from build123d import *

# Parameters (mm, degrees)
SKETCH_13_W                      = 40
SKETCH_13_H                      = 5
SM_BASE_FLANGE_1_DEPTH           = 18
SM_EDGE_FLANGE_1_STRIP_W         = 23.4732
SM_EDGE_FLANGE_1_STRIP_H         = 5
SM_EDGE_FLANGE_1_STRIP_CUT_DEPTH = 40
SM_EDGE_FLANGE_1_DEPTH           = 40
SKETCH_26_R                      = 1.5
CUT_EXTRUDE_1_DEPTH              = 81.956778592
FILLET_1_R                       = 3
SKETCH_32_R                      = 3.3
CUT_EXTRUDE_4_DEPTH              = 1


# Sheet-metal steps are written as plain solids
with BuildPart() as part:
    # 草图13 → 基体-法兰1 (new body)
    with BuildSketch(Plane.XY):
        with Locations((0, -2.5)):
            Rectangle(SKETCH_13_W, SKETCH_13_H)
    extrude(amount=SM_BASE_FLANGE_1_DEPTH)

    # 边线-法兰1 strip (across the edge) → 边线-法兰1 strip cut (cut)
    with BuildSketch(Plane(origin=(-20, 0, 18), x_dir=(0, 0, -1), z_dir=(1, 0, 0))):
        with Locations((-10, -2.5)):
            Rectangle(SM_EDGE_FLANGE_1_STRIP_W, SM_EDGE_FLANGE_1_STRIP_H)
    extrude(amount=SM_EDGE_FLANGE_1_STRIP_CUT_DEPTH, mode=Mode.SUBTRACT)

    # 边线-法兰1 section (across the edge) → 边线-法兰1 (add)
    with BuildSketch(Plane(origin=(-20, 0, 18), x_dir=(0, 0, -1), z_dir=(1, 0, 0))):
        with BuildLine():
            Line((-5, 1.7366), (-5, 70))
            Line((-5, 70), (0, 70))
            Line((0, 70), (0, 1.7366))
            ThreePointArc((0, 1.7366), (0.508638364, 0.508638364), (1.7366, 0))
            Line((1.7366, 0), (1.7366, -5))
            ThreePointArc((1.7366, -5), (-3.026895542, -3.026895542), (-5, 1.7366))
        make_face()
    extrude(amount=SM_EDGE_FLANGE_1_DEPTH)

    # 草图26 → 切除-拉伸1 (cut, through all)
    with BuildSketch(Plane.XZ.offset(5)):
        with Locations(Location((-13.7, 5.5, 0), (0, 0, 270))):
            Circle(SKETCH_26_R)
        with Locations(Location((13.7, 5.5, 0), (0, 0, 270))):
            Circle(SKETCH_26_R)
    extrude(amount=-CUT_EXTRUDE_1_DEPTH, mode=Mode.SUBTRACT)

    # 圆角1
    fillet_1_edges = [part.edges().sort_by_distance(p)[0] for p in [
        (-20, -2.5, 0),
        (20, -2.5, 0),
    ]]
    fillet(fillet_1_edges, radius=FILLET_1_R)

    # 草图32 → 切除-拉伸4 (cut)
    with BuildSketch(Plane(origin=(0, -5, 0), x_dir=(-1, 0, 0), z_dir=(0, -1, 0))):
        with Locations(Location((13.7, -5.5, 0), (0, 0, 90))):
            Circle(SKETCH_32_R)
        with Locations(Location((-13.7, -5.5, 0), (0, 0, 90))):
            Circle(SKETCH_32_R)
    extrude(amount=-CUT_EXTRUDE_4_DEPTH, mode=Mode.SUBTRACT)


solid = part.part
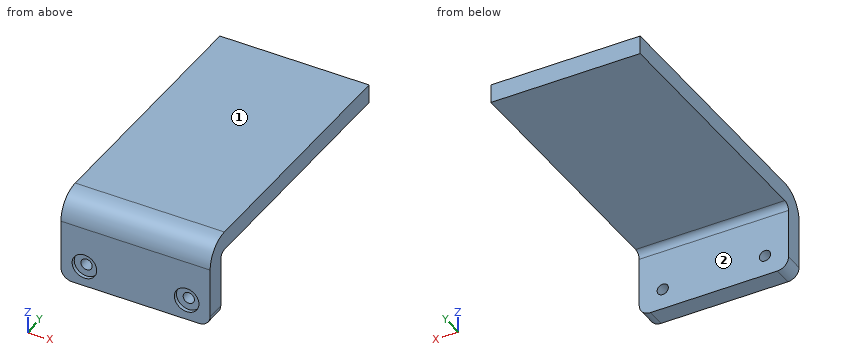
The listing builds one solid part. Answer for the finished solid, in the listing's coordinates (mm). Face numbers are marked on the shaded views. A direction names the side the tool comes from. Coordinates: 2 decimals unless noted, no trailing zeros. Loops run counter-clockwise (first coordinate to the right, second up) from the corner with the lowest first, then second, coordinate; pieces in that order, holes last. Notation, with made-up numbers: (58.25, 59) -> (79.25, 59) arc R16 cw to (79.25, 75) -> close; hole circle Ø6 at (13.5, 29.25). An arc over 180 degrees is marked (long way). Answer in a Markdown table with one row per item. Add a question column.
1. For the marked faces 1 and 2, determine the directions among +Z, -Z, +X, -X, +Y, -Y from which every point of the face is accessible in a straight line to the end or side of a thin tool.
2. The part is cut by section C-C, the plane x = 3. Write down the section's boundary in (y, z), then the cut area to 3 significant figures.
3. The part is cut by section B-B, the plane z = 5.5. Write down the section's boundary in (x, y).
4. The part is cut by section D-D, the plane y = 33.5. Write down the section's boundary in (x, z), then the cut area to 3 significant figures.
5. Flat-ended cylindrical pins translate along their axes: P1, Ø3.5, axis at x = -13.7, z = 5.5, coming from the -Y side; P2, Ø6, axis at x = 13.7, z = 5.5, coming from the +Y side; P3, Ø20, axis at x = 7, y = 36, coming from the -Z side; P4, Ø2.5, axis at x = 13.7, z = 5.5, coming from the +Y side. Find the tip coordinate at first contact, or state that the pin passes through.
6. Consider line 1 (X direction, y = -0.85, z = 5.5); line 2 (X direction, y = -4.25, z = 5.5); line 3 (Z direction, x = 14.5, y = 30). Determine where each line is inside the solid, lowest interval first. Write a range as [from, to].
7. The part is cut by section A-A, the plane x = -13.7. Write down the section's boundary in (y, z), then the cut area to 3 significant figures.
Answer below:
| question | item | result |
|---|---|---|
| 1 | face 1 | +Z, +X, -X, +Y, -Y |
| 1 | face 2 | -Z, +X, -X, +Y |
| 2 | outline | (-5, 0) -> (0, 0) -> (0, 16.26) arc R1.74 cw to (1.74, 18) -> (70, 18) -> (70, 23) -> (1.74, 23) arc R6.74 ccw to (-5, 16.26) -> close |
| 2 | area | 456 mm2 |
| 3 | outline | (-20, -5) -> (-17, -5) -> (-17, -4) -> (-15.2, -4) -> (-15.2, 0) -> (-20, 0) -> close; (-12.2, -4) -> (-10.4, -4) -> (-10.4, -5) -> (10.4, -5) -> (10.4, -4) -> (12.2, -4) -> (12.2, 0) -> (-12.2, 0) -> close; (15.2, -4) -> (17, -4) -> (17, -5) -> (20, -5) -> (20, 0) -> (15.2, 0) -> close |
| 4 | outline | (-20, 18) -> (20, 18) -> (20, 23) -> (-20, 23) -> close |
| 4 | area | 200 mm2 |
| 5 | P1 | y = -4 |
| 5 | P2 | y = 0 |
| 5 | P3 | z = 18 |
| 5 | P4 | through |
| 6 | line 1 | [-20, -15.2], [-12.2, 12.2], [15.2, 20] |
| 6 | line 2 | [-20, -17], [-10.4, 10.4], [17, 20] |
| 6 | line 3 | [18, 23] |
| 7 | outline | (-5, 0) -> (0, 0) -> (0, 4) -> (-4, 4) -> (-4, 2.2) -> (-5, 2.2) -> close; (-5, 8.8) -> (-4, 8.8) -> (-4, 7) -> (0, 7) -> (0, 16.26) arc R1.74 cw to (1.74, 18) -> (70, 18) -> (70, 23) -> (1.74, 23) arc R6.74 ccw to (-5, 16.26) -> close |
| 7 | area | 437 mm2 |
